Autodesk Inventor part; units mm, degrees
ref_plane "YZ Plane" through (0, 0, 0) normal (1, 0, 0) x (0, 1, 0)
ref_plane "XZ Plane" through (0, 0, 0) normal (0, 1, 0) x (-1, 0, 0)
ref_plane "XY Plane" through (0, 0, 0) normal (0, 0, 1) x (1, 0, 0)
sketch "Skizze1" plane through (0, 0, 0) normal (0, 1, 0) x (-1, 0, 0)
  line L0 (3.5, 7.5) -> (-3.5, 7.5)
  line L1 (-3.5, 7.5) -> (-3.5, 2.8284)
  line L2 (-3.5, -7.5) -> (3.5, -7.5)
  line L3 (3.5, -7.5) -> (3.5, -2.8284)
  line L4 (3.5, 7.5) -> (-3.5, -7.5) construction
  line L5 (-3.5, 7.5) -> (3.5, -7.5) construction
  line L6 (-3.5, -2.8284) -> (-3.5, -7.5)
  arc A0 (-3.5, 2.8284) -> (-3.5, -2.8284) centre (0, 0) ccw
  arc A1 (3.5, -2.8284) -> (3.5, 2.8284) centre (0, 0) ccw
  line L7 (3.5, 2.8284) -> (3.5, 7.5)
  line L8 (3.5, -2.8284) -> (3.5, 2.8284) construction
  line L9 (-3.5, -2.8284) -> (-3.5, 2.8284) construction
  arc A2 (-3.5, -2.8284) -> (3.5, -2.8284) centre (0, 0) ccw construction
  arc A3 (3.5, 2.8284) -> (-3.5, 2.8284) centre (0, 0) ccw construction
  dimension "d0" = 7
  dimension "d1" = 15
  dimension "d5" = 4.5
extrude "Extrusion1" add sketch "Skizze1" along normal blind 22
sketch "Skizze2" plane through (0, 0, 0) normal (1, 0, 0) x (0, 1, 0)
  circle A0 centre (15.5, 0) radius 1.5
  line L0 (0, -7.5) -> (22, -7.5)
  line L1 (22, -2.8284) -> (22, 2.8284)
  point P0 (0, 0)
  dimension "d8" = 3
  dimension "d9" = 7.5
  dimension "d10" = 6.5
extrude "Extrusion2" cut sketch "Skizze2" along normal through all both and the other way through all
properties part number "simpleste Anbindung"
Can you work these out from the model? Positions are in its coordinate system, mm. A direction names the side the tool comes from. Coordinates: 2 decimals unless noted, no trailing zeros. Write each loop counter-clockwise with the first axis right and the second up, starting at its lowest first coordinate (ties: lowest second). Pieces come first, ordered by that corner, then holes. Notation, with made-up numbers: (-26, 10.5) - (4, 10.5) arc R10 cw to (4, 20.5) - close; hole circle Ø7 at (31.5, -20). An arc over 180 degrees is marked (long way). Return JSON: item names as keys, results as strings. Group by question number.
Item 1: Which directions (+Z, -Z, +X, -X, +Y, -Y) give clear straight access to the entire face, cutting with the end or side of a thin tool? Please do faces 5 (the face through (-3.5, 11, -5)), 6 (the face through (3.5, 11, 5)), 7 (the face through (3.5, 11, -5)).
Item 2: I'm going to push flat-ended pins straight in: pin 1 Ø2.5 at (y, z) = (9, 5) entering from -X; pin 2 Ø1.4 at (y, z) = (7, -4) entering from +X. Where does each tip first touch, or does it pass through?
Item 3: We'd pull the mould along Y, two halves only. Please class faces 1 (the face through (0, 22, 0)), 2 (the face through (0, 0, 0)), 3 (the face through (0, 14, 0)), 4 (the face through (-3.5, 11, 5)): pulls with the +Y half, pulls with the -Y half, needs draft (parallel to the pull), parting line crosses it, or undercut.
Item 4: If we section it at D-D (z = -5): Write out the boundary of the cut face in (x, y), then the cut area to 3 significant figures.
Item 5: If we section it at A-A (z = 0): Write out the boundary of the cut face in (x, y).
Item 6: Please list where these lines run through material, in increasing order: probe 1 along Z at (x, y) = (-3, 15.5); probe 2 along Y at (x, z) = (1.25, 0); probe 3 along X at (y, z) = (14, -5.75).
Item 7: If we section it at C-C (y = 16.75): Write out the boundary of the cut face in (x, z), then the cut area to 3 significant figures.
Item 8: If we section it at B-B (x = -3.25): Write out the boundary of the cut face in (y, z).
Return value:
{
 "1": {"face 5": "-Z, -X, +Y, -Y", "face 6": "+Z, +X, +Y, -Y", "face 7": "-Z, +X, +Y, -Y"},
 "2": {"pin 1": "stops at x = -3.5", "pin 2": "stops at x = 3.5"},
 "3": {"face 1": "pulls with the +Y half", "face 2": "pulls with the -Y half", "face 3": "undercut", "face 4": "needs draft"},
 "4": {"outline": "(-3.5, 0) - (3.5, 0) - (3.5, 22) - (-3.5, 22) - close", "area": "154 mm^2"},
 "5": {"outline": "(-4.5, 0) - (4.5, 0) - (4.5, 14) - (-4.5, 14) - close; (-4.5, 17) - (4.5, 17) - (4.5, 22) - (-4.5, 22) - close"},
 "6": {"probe 1": "z = -7.5 to -1.5, 1.5 to 7.5", "probe 2": "y = 0 to 14, 17 to 22", "probe 3": "x = -3.5 to 3.5"},
 "7": {"outline": "(-4.42, -0.83) arc R4.5 ccw to (-3.5, -2.83) - (-3.5, -7.5) - (3.5, -7.5) - (3.5, -2.83) arc R4.5 ccw to (4.42, -0.83) - close; (-4.42, 0.83) - (4.42, 0.83) arc R4.5 ccw to (3.5, 2.83) - (3.5, 7.5) - (-3.5, 7.5) - (-3.5, 2.83) arc R4.5 ccw to start", "area": "97.9 mm^2"},
 "8": {"outline": "(0, -7.5) - (22, -7.5) - (22, 7.5) - (0, 7.5) - close; hole circle Ø3 at (15.5, 0)"}
}
